```python
from build123d import *

# Parameters (mm, degrees)
F1_DEPTH    = 50
F2_T1_DEPTH = 57.9983578358


# Not quite as in the source:
# - a fillet or chamfer that OpenCascade refuses, or shapes differently, is made with other operations: its cross-section is extruded or revolved along the edge and cut away or added


with BuildPart() as f1:
    # F0 (on Front) → F1 (new body)
    with BuildSketch(Plane.XZ):
        with BuildLine():
            Line((7.5, 5), (0, 5))
            Line((0, 5), (-7.5, 5))
            Line((-7.5, 5), (-7.5, 0))
            Line((-7.5, 0), (-2.5, 0))
            ThreePointArc((-2.5, 0), (-1.767766953, 1.767766953), (0, 2.5))
            ThreePointArc((0, 2.5), (1.767766953, 1.767766953), (2.5, 0))
            Line((2.5, 0), (7.5, 0))
            Line((7.5, 0), (7.5, 5))
        make_face()
    extrude(amount=F1_DEPTH)

    # F2: chamfer of 2 on 2 edges, made by hand

    # F2_s2 → F2_t1 (cut)
    with BuildSketch(Plane.XZ.offset(-3.9991789179)):
        with BuildLine():
            Line((-4.0311288741, 0), (-2.2395160412, 1.1111111111))
            ThreePointArc((-2.2395160412, 1.1111111111), (-2.4271314798, 0.5991934409), (-2.5, 0))
            Line((-2.5, 0), (-4.0311288741, 0))
        make_face()
        with BuildLine():
            Line((4.0311288741, 0), (2.2395160412, 1.1111111111))
            ThreePointArc((2.2395160412, 1.1111111111), (2.4271314798, 0.5991934409), (2.5, 0))
            Line((2.5, 0), (4.0311288741, 0))
        make_face()
    extrude(amount=F2_T1_DEPTH, mode=Mode.SUBTRACT)


solid = f1.part
```
Work out the finished part from the listing and answer in its coordinate system (mm). A direction names the side the tool comes from. Coordinates: 2 decimals unless noted, no trailing zeros. Write each loop counter-clockwise with the first axis right and the second up, starting at its lowest first coordinate (ties: lowest second). Pieces come first, ordered by that corner, then holes.
Q1. A cutting plane is placed at A-A, the plane y = -34. Give the vertices of the cut face in (x, z).
Q2. Determine the mould class of faces 1 (the face through (-7.5, -25, 3)), 2 (the face through (-3.148, -24.65, 0.548)), 3 (the face through (0, -50, 3)) for opening direction X: released by +X, released by -X, zero draft, split by the parting line, or undercut.
Q3. A cutting plane is placed at B-B, the plane x = 1.5. Give the vertices of the cut face in (y, z).
Q4. Which of the six approach directions +Z, -Z, +X, -X, +Y, -Y give full straight-line access (tool end or side, diameter ignored) to faces 4 (the face through (0, 0, 3)), 5 (the face through (3.148, -24.65, 0.548))?
Q5. Find the intervals of material crossed by line 1 (X direction, y = -15.5, z = 1.45); line 2 (X direction, y = -10, z = 0.65); line 3 (Z direction, x = 3.5, y = -41.5), in increasing order.
Findings below:
1. outline: (-7.5, 0) - (-4.03, 0) - (-2.24, 1.11) arc R2.5 cw to (2.24, 1.11) - (4.03, 0) - (7.5, 0) - (7.5, 5) - (-7.5, 5) - close
2. face 1: released by -X
2. face 2: undercut
2. face 3: zero draft
3. outline: (-50, 2) - (0, 2) - (0, 5) - (-50, 5) - close
4. face 4: +Z, -Z, +X, -X, +Y
4. face 5: -Z, +Y, -Y
5. line 1: x = -7.5 to -2.04, 2.04 to 7.5
5. line 2: x = -7.5 to -2.98, 2.98 to 7.5
5. line 3: z = 0.33 to 5
